Job drawing, mm, ordinate dimensions from the low corner. One solid piece. A direction names the side the tool comes from. Round coordinates to 2 decimals unless told otherwise and drop trailing zeros. Write each loop counter-clockwise with the first axis right and the second up, starting at its lowest first coordinate (ties: lowest second). Pieces come first, ordered by that corner, then holes. Notation, with made-up numbers: (-13.5, 5) - (39.5, 5) arc R35 cw to (39.5, 42) - close; hole circle Ø11 at (-5, -29). An arc over 180 degrees is marked (long way). Write each question's results on one line, items separated by ' | '.
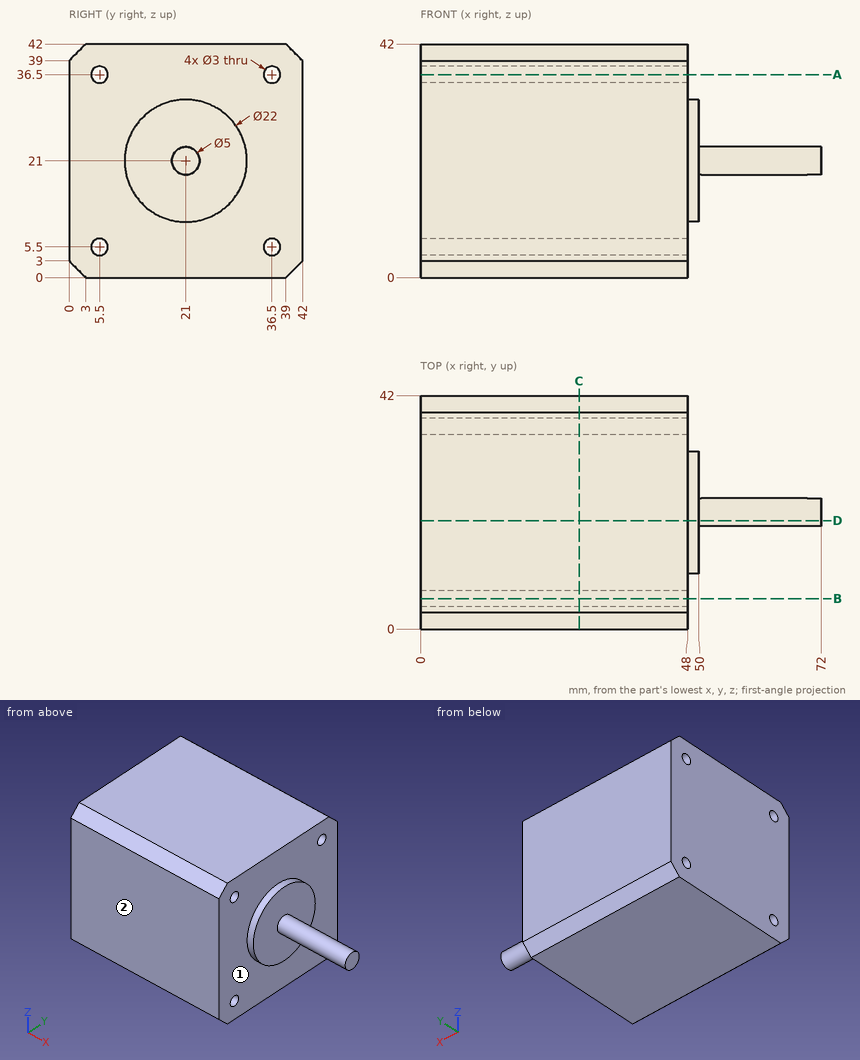
(1) Slice it at A-A, the plane z = 36.5. Write the cut outline in (x, y), and give its area (3 significant figures).
Worked answers:
outline: (0, 0) - (48, 0) - (48, 4) - (0, 4) - close; (0, 7) - (48, 7) - (48, 35) - (0, 35) - close; (0, 38) - (48, 38) - (48, 42) - (0, 42) - close | area: 1,730 mm2
(2) Tool access for the marked faces 1 and 2: list every direction of +Z, -Z, +X, -X, +Y, -Y with a clear straight run to the whole face (end or side of a thin tool).
Worked answers:
face 1: +X | face 2: +Z, -Z, +X, -X, -Y
(3) Drill centre lines: probe 1 along Z at (x, y) = (33, 36.5); probe 2 along Y at (x, z) = (38, 36). Where is each one in solid material? Low to high. Write a range as [from, to].
Worked answers:
probe 1: z = [0, 4], [7, 35], [38, 42] | probe 2: y = [0, 4.09], [6.91, 35.09], [37.91, 42]
(4) Flat gauge pins, fed straight in: pin 1 Ø2.5 at (y, z) = (5.5, 5.5) entering from -X; pin 2 Ø12 at (y, z) = (33, 14) entering from +X; pin 3 Ø2 at (y, z) = (6.5, 23) entering from +X. Where does each tip first touch, or does it go through?
Worked answers:
pin 1: passes through | pin 2: stops at x = 50 | pin 3: stops at x = 48
(5) Slice it at D-D, the plane y = 19.5. Write the cut outline in (x, z).
Worked answers:
outline: (0, 0) - (48, 0) - (48, 10.1) - (50, 10.1) - (50, 19) - (72, 19) - (72, 23) - (50, 23) - (50, 31.9) - (48, 31.9) - (48, 42) - (0, 42) - close
(6) Slice it at C-C, the plane x = 28.5. Write the cut outline in (y, z).
Worked answers:
outline: (0, 3) - (3, 0) - (39, 0) - (42, 3) - (42, 39) - (39, 42) - (3, 42) - (0, 39) - close; hole circle Ø3 at (5.5, 5.5); hole circle Ø3 at (5.5, 36.5); hole circle Ø3 at (36.5, 5.5); hole circle Ø3 at (36.5, 36.5)
